Part print with two shaded views. Sizes in mm from the minimum x, y, z corner. A direction names the side the tool comes from. Round coordinates to 2 decimals unless told otherwise and drop trailing zeros. Loops run counter-clockwise (first coordinate to the right, second up) from the corner with the lowest first, then second, coordinate; pieces in that order, holes last.
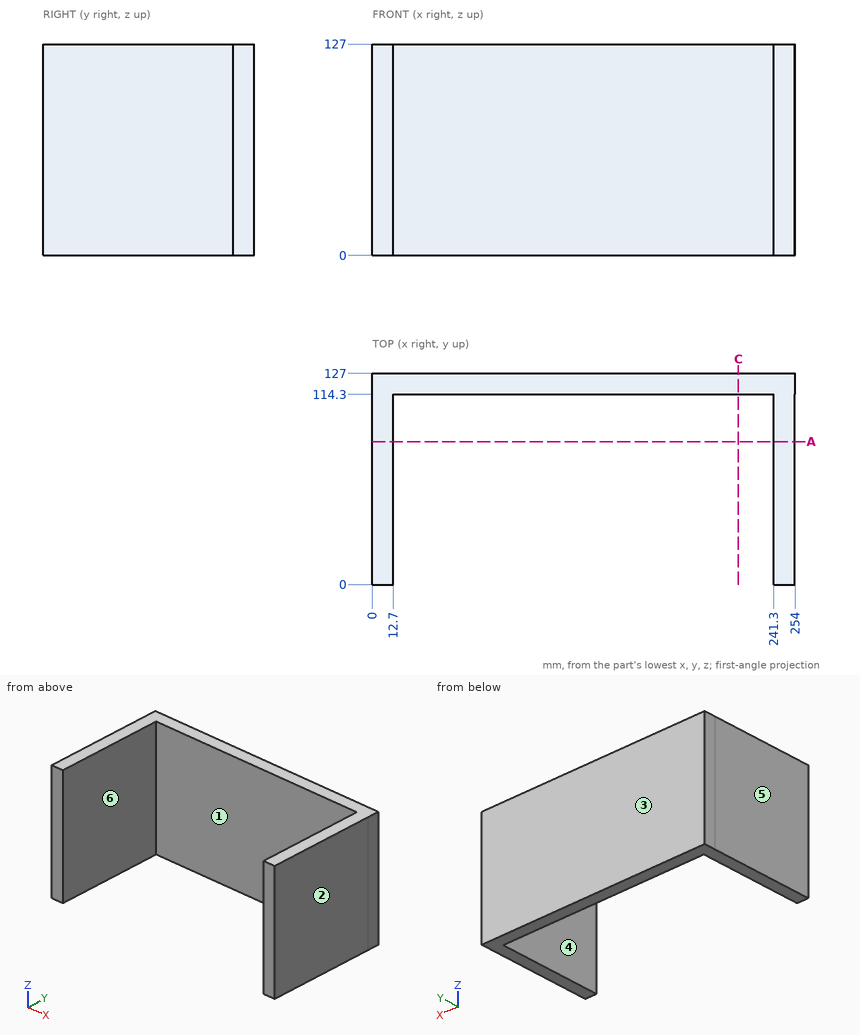
Item 1: 3-axis set-ups, long thin cutter, end or side, ignore diameter. For the marked faces 5 and 6: which of +Z, -Z, +X, -X, +Y, -Y reach the whole face in a straight line?
Verdict:
face 5: +Z, -Z, -X, +Y, -Y
face 6: +Z, -Z, -Y
Item 2: Wall check: L1, parallel to X at y = 49.5, z = 76; L2, parallel to Y at x = 74, z = 21.5. Give the ranges that are in metal, low to high.
Verdict:
L1: x = 0 to 12.7, 241.3 to 254
L2: y = 114.3 to 127
Item 3: Cut at C-C (x = 220). List the corners of the cut face in (y, z).
Verdict:
outline: (114.3, 0) - (127, 0) - (127, 127) - (114.3, 127) - close
Item 4: Cut at A-A (y = 86). List the corners of the cut face in (x, z), plus the area to 3 significant figures.
Verdict:
outline: (0, 0) - (12.7, 0) - (12.7, 127) - (0, 127) - close; (241.3, 0) - (254, 0) - (254, 127) - (241.3, 127) - close
area: 3,230 mm2
Item 5: Flat gauge pin, fed straight in: P1, Ø3, axis at x = 63, z = 104.5, coming from the -Y side. Where does the tip first touch, or does it go through?
Verdict:
P1: stops at y = 114.3
Item 6: Mould opens along X. For the marked faces 1, 2, 3 and 4 say: released by +X, released by -X, zero draft, split by the parting line, or undercut.
Verdict:
face 1: undercut
face 2: released by +X
face 3: zero draft
face 4: undercut
